Part model, mm, in its own coordinate system. A direction names the side the tool comes from. Give positions to 0.01 mm unless a question says otherwise; leave off trailing zeros. Loops run counter-clockwise (first coordinate to the right, second up) from the corner with the lowest first, then second, coordinate; pieces in that order, holes last. Notation, with made-up numbers: M 58,-19 L 66,-19 A20 ccw 66,-13 Z; hole C 10,57 d6. An arc over 180 degrees is marked long. Answer in a Markdown table with one row per item.
from build123d import *

# Parameters (mm, degrees)
ESQUISSE1_W             = 30
ESQUISSE1_H             = 37.5
BOSS_EXTRU_1_DEPTH      = 35
ESQUISSE2_R             = 14
BOSS_EXTRU_2_DEPTH      = 8
ESQUISSE3_R             = 11.8
BOSS_EXTRU_3_DEPTH      = 6
ESQUISSE4_R             = 14
BOSS_EXTRU_4_DEPTH      = 14
ESQUISSE5_R             = 11.5
BOSS_EXTRU_5_DEPTH      = 8
ENL_V_MAT_EXTRU_1_DEPTH = 20
ESQUISSE9_W             = 9.8
ESQUISSE9_H             = 37.1
ENL_V_MAT_EXTRU_2_DEPTH = 0.2


with BuildPart() as part:
    # Esquisse1 → Boss.-Extru.1 (new body)
    with BuildSketch(Plane.XY):
        Rectangle(ESQUISSE1_W, ESQUISSE1_H)
    extrude(amount=BOSS_EXTRU_1_DEPTH)

    # Esquisse2 → Boss.-Extru.2 (add)
    with BuildSketch(Plane.XY.offset(35)):
        Circle(ESQUISSE2_R)
    extrude(amount=BOSS_EXTRU_2_DEPTH)

    # Esquisse3 → Boss.-Extru.3 (add)
    with BuildSketch(Plane.XY.offset(43)):
        Circle(ESQUISSE3_R)
    extrude(amount=BOSS_EXTRU_3_DEPTH)

    # Esquisse4 → Boss.-Extru.4 (add)
    with BuildSketch(Plane.XY.offset(49)):
        Circle(ESQUISSE4_R)
    extrude(amount=BOSS_EXTRU_4_DEPTH)

    # Esquisse5 → Boss.-Extru.5 (add)
    with BuildSketch(Plane.XY.offset(63)):
        Circle(ESQUISSE5_R)
    extrude(amount=BOSS_EXTRU_5_DEPTH)

    # Esquisse7 → Révolution1 (revolve)
    with BuildSketch(Plane(origin=(0, 0, 0), x_dir=(1, 0, 0), z_dir=(0, 1, 0))):
        with BuildLine():
            Line((0, -71), (12.5, -71))
            Line((12.5, -71), (12.5, -72))
            Line((12.5, -72), (18.5, -72))
            Line((18.5, -72), (18.5, -71))
            Line((18.5, -71), (19.5, -71))
            Line((19.5, -71), (19.5, -76))
            ThreePointArc((19.5, -76), (9.801147892, -77.498691947), (0, -78))
            Line((0, -78), (0, -71))
        make_face()
    revolve(axis=Axis((0, 0, 71), (0, 0, -1)))

    # Esquisse8 → Enlèv. mat.-Extru.1 (cut)
    with BuildSketch(Plane(origin=(0, 0, 0), x_dir=(-1, 0, 0), z_dir=(0, 0, -1))):
        Polygon((-5, 18.75), (-5, 18.55), (-14.8, 18.55), (-14.8, -18.55), (-5, -18.55), (-5, -18.75), (-15, -18.75), (-15, 18.75), align=None)
        Polygon((14.8, -18.55), (5, -18.55), (5, -18.75), (15, -18.75), (15, 18.75), (5, 18.75), (5, 18.55), (14.8, 18.55), align=None)
    extrude(amount=-ENL_V_MAT_EXTRU_1_DEPTH, mode=Mode.SUBTRACT)

    # Esquisse9 → Enlèv. mat.-Extru.2 (cut)
    with BuildSketch(Plane(origin=(0, 0, 0), x_dir=(-1, 0, 0), z_dir=(0, 0, -1))):
        with Locations((-9.9, 0)):
            Rectangle(ESQUISSE9_W, ESQUISSE9_H)
        with Locations((9.9, 0)):
            Rectangle(ESQUISSE9_W, ESQUISSE9_H)
    extrude(amount=-ENL_V_MAT_EXTRU_2_DEPTH, mode=Mode.SUBTRACT)


solid = part.part
(1) Which spindle directions (+Z, -Z, +X, -X, +Y, -Y) get a long thin tool onto all of the face, cutting with end or side? Do faces 5 (the face through (0, 18.75, 21)), 6 (the face through (10, 18.55, 10)), 7 (the face through (12.932, -5.362, 38.944)). Say none if no direction does.
Recorded:
| item | result |
|---|---|
| face 5 | -Z, +X, -X, +Y |
| face 6 | -Z, +X, +Y |
| face 7 | none |
(2) Saw through at B-B (z = 11). Write the cut outline in (x, y), plus the area to 3 significant figures.
Recorded:
| item | result |
|---|---|
| outline | M -14.8,-18.55 L -5,-18.55 L -5,-18.75 L 5,-18.75 L 5,-18.55 L 14.8,-18.55 L 14.8,18.55 L 5,18.55 L 5,18.75 L -5,18.75 L -5,18.55 L -14.8,18.55 Z |
| area | 1,100 mm^2 |
(3) Pin check, flat tips, straight feed: pin 1 Ø12.5 at (x, y) = (2.5, 3) entering from -Z; pin 2 Ø8 at (x, y) = (13, -12) entering from -Z; pin 3 Ø7.5 at (y, z) = (2, 28) entering from -X; pin 4 Ø16 at (y, z) = (2.5, 9) entering from +X. Stop position of each tip, or through.
Recorded:
| item | result |
|---|---|
| pin 1 | stops at z = 0 |
| pin 2 | stops at z = 0.2 |
| pin 3 | stops at x = -15 |
| pin 4 | stops at x = 14.8 |
(4) Drill centre lines: line 1 along Y through (x, z) = (0, 71.5); line 2 along Z through (x, y) = (-11.5, 4.5). Where is each one in solid material? Low to high.
Recorded:
| item | result |
|---|---|
| line 1 | y = -19.5 to -18.5, -12.5 to 12.5, 18.5 to 19.5 |
| line 2 | z = 0.2 to 43, 49 to 63, 71 to 77.2 |
(5) Saw through at C-C (z = 45.5). Write the cut outline in (x, y), plus the area to 3 significant figures.
Recorded:
| item | result |
|---|---|
| outline | C 0,0 d23.6 |
| area | 437 mm^2 |
(6) Pull direction Y, two halves, no side cores. Call faces 1 (the face through (-1.5, 11.4, 66.9)), 2 (the face through (11.923, -3.755, 71.507)), 3 (the face through (2, 11.5, 63)), 4 (the face through (-12.1, 3.9, 72)): +Y half, -Y half, draft (parallel to the pull), parting line (faces both ways), or undercut.
Recorded:
| item | result |
|---|---|
| face 1 | parting line |
| face 2 | undercut |
| face 3 | draft |
| face 4 | undercut |
